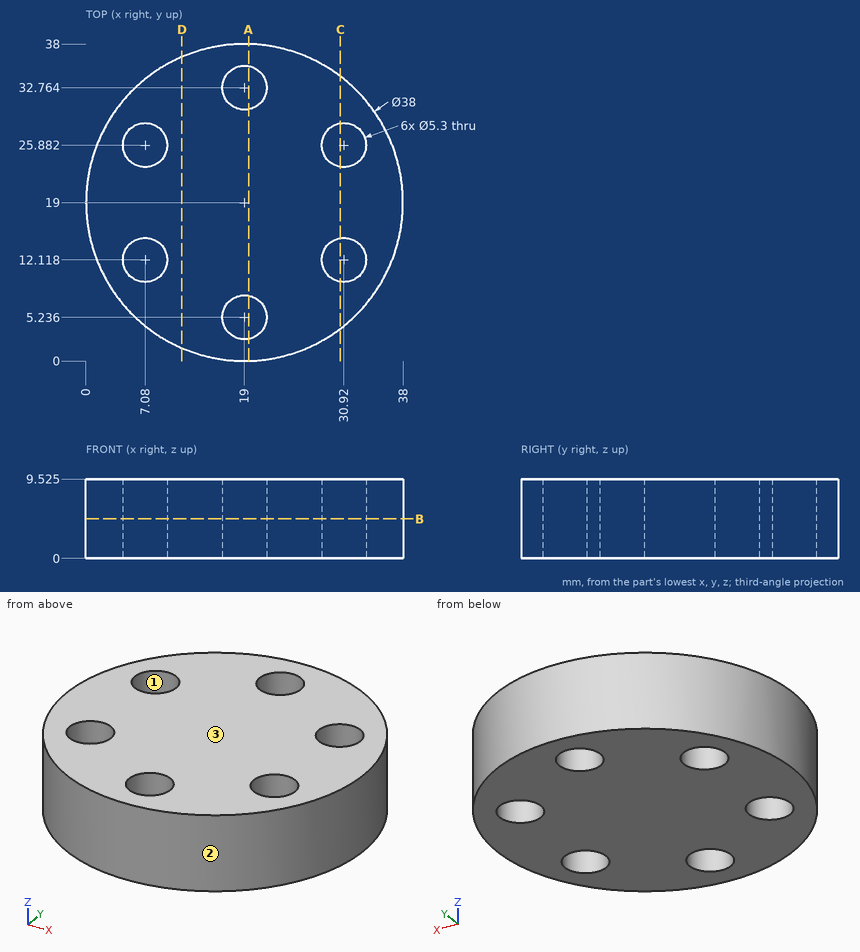
Part print with two shaded views. Sizes in mm from the minimum x, y, z corner. Coordinates: 2 decimals unless noted, no trailing zeros. Write each loop counter-clockwise with the first axis right and the second up, starting at its lowest first coordinate (ties: lowest second). Pieces come first, ordered by that corner, then holes.
1. Band-saw the part on D-D, the plane x = 11.5. Give the cut face in (y, z) (1 decimal).
Answer block:
outline: (1.5, 0) - (36.5, 0) - (36.5, 9.5) - (1.5, 9.5) - close
2. Pull direction Y, two halves, no side cores. Call the marked faces 1, 2 and 3: released by +Y, released by -Y, zero draft, split by the parting line, or undercut.
Answer block:
face 1: undercut
face 2: split by the parting line
face 3: zero draft
3. Band-saw the part on B-B, the plane z = 4.75. Give the cut face in (x, y), and give its area (3 significant figures).
Answer block:
outline: circle Ø38 at (19, 19); hole circle Ø5.3 at (7.08, 12.12); hole circle Ø5.3 at (7.08, 25.88); hole circle Ø5.3 at (19, 5.24); hole circle Ø5.3 at (19, 32.76); hole circle Ø5.3 at (30.92, 12.12); hole circle Ø5.3 at (30.92, 25.88)
area: 1,000 mm2
4. Drill centre lines: probe 1 along X at (y, z) = (27.5, 8); probe 2 along Y at (x, z) = (33, 1.5) (1 decimal); probe 3 along X at (y, z) = (23.5, 7.75). Where is each one in solid material? Low to high.
Answer block:
probe 1: x = 2.01 to 4.98, 9.18 to 28.82, 33.02 to 35.99
probe 2: y = 6.2 to 10.5, 13.8 to 24.2, 27.5 to 31.8
probe 3: x = 0.54 to 5.92, 8.24 to 29.76, 32.08 to 37.46
5. Drop flat-ended pins along their axis: pin 1 (1.5 mm diameter, centred on x = 17, y = 30.5, fed in from -Z); pin 2 (3 mm diameter, centred on y = 23.5, z = 7.5, fed in from -X); pin 3 (1.5 mm diameter, centred on y = 25, z = 5, fed in from -X); pin 4 (4 mm diameter, centred on x = 19, y = 32.76, fed in from +Z). Give the stop position or say it passes through.
Answer block:
pin 1: stops at z = 0
pin 2: stops at x = 0.24
pin 3: stops at x = 0.74
pin 4: passes through
6. Band-saw the part on A-A, the plane x = 19.5. Give the cut face in (y, z) (1 decimal).
Answer block:
outline: (0, 0) - (2.6, 0) - (2.6, 9.5) - (0, 9.5) - close; (7.8, 0) - (30.2, 0) - (30.2, 9.5) - (7.8, 9.5) - close; (35.4, 0) - (38, 0) - (38, 9.5) - (35.4, 9.5) - close
7. Band-saw the part on C-C, the plane x = 30.5. Give the cut face in (y, z) (1 decimal), and give its area (3 significant figures).
Answer block:
outline: (3.9, 0) - (9.5, 0) - (9.5, 9.5) - (3.9, 9.5) - close; (14.7, 0) - (23.3, 0) - (23.3, 9.5) - (14.7, 9.5) - close; (28.5, 0) - (34.1, 0) - (34.1, 9.5) - (28.5, 9.5) - close
area: 188 mm2
